Geometry check sheet. Reference: drawing and pictorial views, mm from the part's lowest x, y, z. A direction names the side the tool comes from. Round coordinates to 2 decimals unless told otherwise and drop trailing zeros. Write each loop counter-clockwise with the first axis right and the second up, starting at its lowest first coordinate (ties: lowest second). Pieces come first, ordered by that corner, then holes. Notation, with made-up numbers: (13, -38) -> (35, -38) arc R36 cw to (35, -3) -> close; hole circle Ø4 at (34, -37). An arc over 180 degrees is marked (long way). Answer as a JSON object with one key per item and string values. Group by question number.
(1) Gauge pin test, flat end, axial feed: pin 1 Ø12 at (x, z) = (11, 10) entering from +Y. Record the tip position at first contact, or that the pin passes through.
(2) Draft check along X on the marked faces 1, 2 and 3. Enter one of: released by +X, released by -X, zero draft, split by the parting line, or undercut.
(3) Sectioned sample at B-B on y = 11.25. Record the cut outline in (x, z), and give its area (3 significant figures).
(4) Set-up check for the marked faces 4 and 5: record each of +Z, -Z, +X, -X, +Y, -Y from which the full face is reachable in a straight line by a thin tool's end or side.
(5) Sectioned sample at A-A on z = 13.5. Record the cut outline in (x, y), and give its area (3 significant figures).
(6) Sectioned sample at C-C on x = 12.75. Record the cut outline in (y, z), and give its area (3 significant figures).
(7) Scan line: L1, parallel to Z at x = 3, y = 15. Record every from-to range of solid material in increasing order. Write a range as from..to.
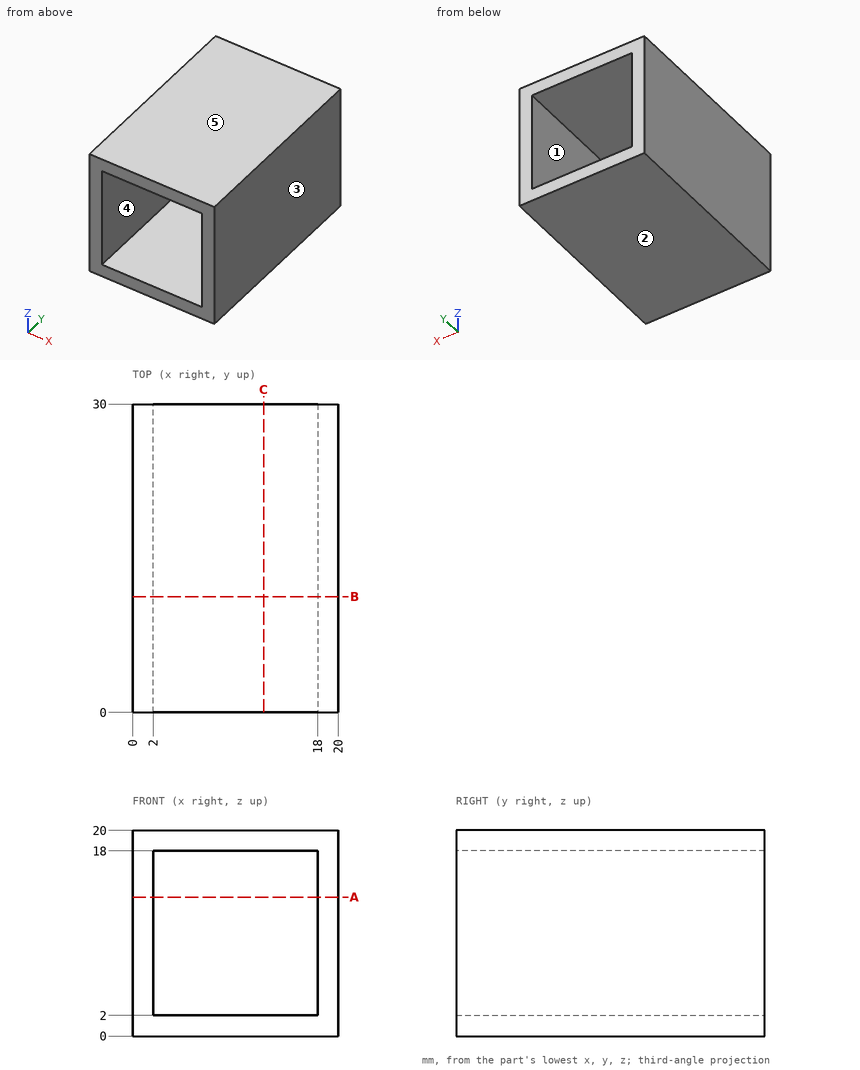
Computed values:
{
 "1": {"pin 1": "through"},
 "2": {"face 1": "undercut", "face 2": "zero draft", "face 3": "released by +X"},
 "3": {"outline": "(0, 0) -> (20, 0) -> (20, 20) -> (0, 20) -> close; hole (2, 2) -> (18, 2) -> (18, 18) -> (2, 18) -> close", "area": "144 mm2"},
 "4": {"face 4": "+Y, -Y", "face 5": "+Z, +X, -X, +Y, -Y"},
 "5": {"outline": "(0, 0) -> (2, 0) -> (2, 30) -> (0, 30) -> close; (18, 0) -> (20, 0) -> (20, 30) -> (18, 30) -> close", "area": "120 mm2"},
 "6": {"outline": "(0, 0) -> (30, 0) -> (30, 2) -> (0, 2) -> close; (0, 18) -> (30, 18) -> (30, 20) -> (0, 20) -> close", "area": "120 mm2"},
 "7": {"L1": "0..2, 18..20"}
}
